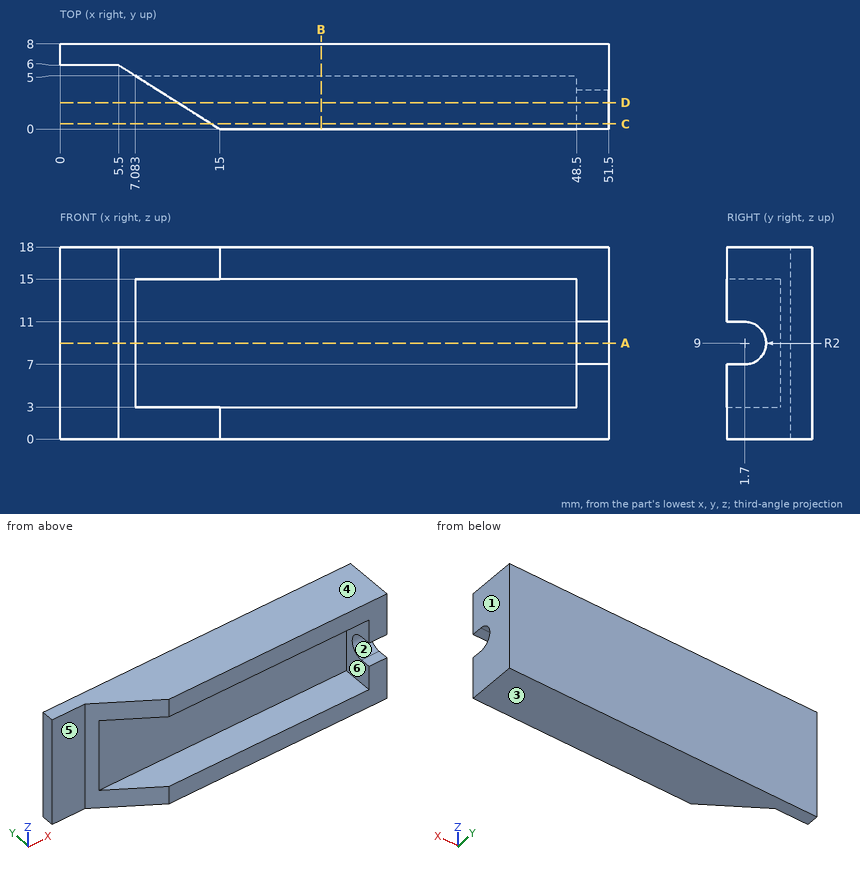
The drawing under review shows one solid part. Ordinate dimensions are in mm from its lowest x, y, z. A direction names the side the tool comes from. Round coordinates to 2 decimals unless told otherwise and drop trailing zeros. Write each loop counter-clockwise with the first axis right and the second up, starting at its lowest first coordinate (ties: lowest second). Pieces come first, ordered by that corner, then holes. Notation, with made-up numbers: (28.5, 26) - (48.5, 26) arc R8 ccw to (48.5, 39) - close; hole circle Ø6 at (13, 27). An arc over 180 degrees is marked (long way). Put each result on its own line as item: value.
Q1. We need section C-C (y = 0.5). Give the boundary of the cut face in (x, z), and give its area (3 significant figures).
Solved:
outline: (14.21, 0) - (51.5, 0) - (51.5, 7) - (48.5, 7) - (48.5, 3) - (14.21, 3) - close; (14.21, 15) - (48.5, 15) - (48.5, 11) - (51.5, 11) - (51.5, 18) - (14.21, 18) - close
area: 248 mm2
Q2. We need section B-B (x = 24.5). Give the boundary of the cut face in (y, z), and give its area (3 significant figures).
Solved:
outline: (0, 0) - (8, 0) - (8, 18) - (0, 18) - (0, 15) - (5, 15) - (5, 3) - (0, 3) - close
area: 84.0 mm2
Q3. We need section A-A (z = 9). Give the boundary of the cut face in (x, y).
Solved:
outline: (0, 6) - (5.5, 6) - (7.08, 5) - (48.5, 5) - (48.5, 3.7) - (51.5, 3.7) - (51.5, 8) - (0, 8) - close
Q4. Wall thickness on probe 1 along Z at (x, y) = (26.5, 0.5); probe 2 along Y at (x, z) = (30, 12); probe 3 along X at (y, z) = (3.5, 7): over which ranges is each line inside the solid? List them lowest first.
Solved:
probe 1: z = 0 to 3, 15 to 18
probe 2: y = 5 to 8
probe 3: x = 48.5 to 51.5
Q5. Insertion check: pin 1 Ø6 at (x, z) = (2, 10) entering from -Y; pin 2 Ø1.5 at (x, y) = (7.5, 3) entering from +Z. Each pin has a flat end and moves straight along its axis. Give the tip position at first contact, or say it passes through.
Solved:
pin 1: stops at y = 6
pin 2: passes through
Q6. Machinability: for the marked faces 4, 5 and 6, which of the approach directions +Z, -Z, +X, -X, +Y, -Y give a long, thin tool a straight path to every point of the face, cutting with its end or side? Answer none if there is none.
Solved:
face 4: +Z, +X, -X, +Y, -Y
face 5: +Z, -Z, -X, -Y
face 6: -X, -Y
Q7. Mouldability with a two-part tool opening along Z and no side actions: class the marked faces 1, 2 and 3 as released by +Z, released by -Z, zero draft, split by the parting line, or undercut.
Solved:
face 1: zero draft
face 2: undercut
face 3: released by -Z
Q8. We need section D-D (y = 2.5). Give the boundary of the cut face in (x, z).
Solved:
outline: (11.04, 0) - (51.5, 0) - (51.5, 7.17) - (48.5, 7.17) - (48.5, 3) - (11.04, 3) - close; (11.04, 15) - (48.5, 15) - (48.5, 10.83) - (51.5, 10.83) - (51.5, 18) - (11.04, 18) - close
